The listing builds one solid part. Answer for the finished solid, in the listing's coordinates (mm). Give positions to 0.01 mm unless a question says otherwise; leave off trailing zeros. Loops run counter-clockwise (first coordinate to the right, second up) from the corner with the lowest first, then second, coordinate; pieces in that order, holes last.
Item 1: Section A-A, the plane z = 117.5 is taken. Give the vertices of the cut face in (x, y).
Item 2: Section B-B, the plane y = -10.5 is taken. Give the vertices of the cut face in (x, z).
Item 3: Consider line 1 along Z through (x, y) = (0, -4.75); line 2 along X through (y, z) = (3.5, 238). Determine where each line is inside the solid, lowest interval first.
Item 4: Each of these flat-tipped pins is pushed along its axis until it touches: pin 1 Ø2.5 at (x, y) = (0.5, -2) entering from -Z; pin 2 Ø5 at (x, y) = (10, -6) entering from -Z; pin 3 Ø1 at (x, y) = (1, -6) entering from +Z; pin 4 Ø3 at (x, z) = (0, 5) entering from +Y. Where does it stop, or does it pass through?
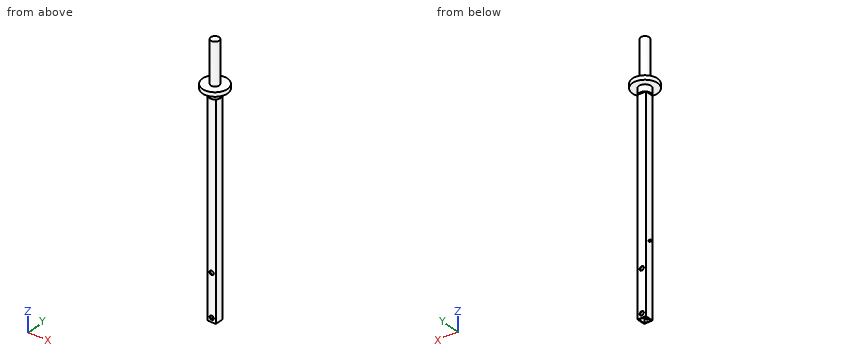
from build123d import *

# Parameters (mm, degrees)
SKETCH_W     = 10
SKETCH_H     = 10
SKETCH_W_2   = 8
SKETCH_H_2   = 8
PAD_DEPTH    = 250
SKETCH001_R  = 2.5
POCKET_DEPTH = 10.001
SKETCH002_R  = 1
PAD001_DEPTH = 2
SKETCH003_R  = 7.071068
PAD002_DEPTH = 8
SKETCH004_R  = 15
PAD003_DEPTH = 5
SKETCH005_R  = 5
PAD004_DEPTH = 50


with BuildPart() as part:
    # Sketch → Pad (new body)
    with BuildSketch(Plane.XY):
        Rectangle(SKETCH_W, SKETCH_H)
        Rectangle(SKETCH_W_2, SKETCH_H_2, mode=Mode.SUBTRACT)
    extrude(amount=PAD_DEPTH)

    # Sketch001 (on Face3 of Pad) → Pocket (cut, through all)
    with BuildSketch(Plane.XZ.offset(5)):
        with Locations((0, 5)):
            Circle(SKETCH001_R)
        with Locations((0, 55)):
            Circle(SKETCH001_R)
    extrude(amount=-POCKET_DEPTH, mode=Mode.SUBTRACT)

    # Sketch002 (on Face2 of Pocket) → Pad001 (join)
    with BuildSketch(Plane(origin=(-5, 0, 0), x_dir=(0, -1, 0), z_dir=(-1, 0, 0))):
        with Locations((0, 86)):
            Circle(SKETCH002_R)
    extrude(amount=PAD001_DEPTH)

    # Sketch003 (on Face4 of Pad001) → Pad002 (join)
    with BuildSketch(Plane.XY.offset(250)):
        Circle(SKETCH003_R)
    extrude(amount=PAD002_DEPTH)

    # Sketch004 (on Face6 of Pad002) → Pad003 (join)
    with BuildSketch(Plane.XY.offset(258)):
        Circle(SKETCH004_R)
    extrude(amount=PAD003_DEPTH)

    # Sketch005 (on Face3 of Pad003) → Pad004 (join)
    with BuildSketch(Plane.XY.offset(263)):
        Circle(SKETCH005_R)
    extrude(amount=PAD004_DEPTH)


solid = part.part
Worked answers:
1. outline: (-5, -5) - (5, -5) - (5, 5) - (-5, 5) - close; hole (-4, -4) - (4, -4) - (4, 4) - (-4, 4) - close
2. outline: (-10.71, 258) - (10.71, 258) - (10.71, 263) - (-10.71, 263) - close
3. line 1: z = 0 to 2.5, 7.5 to 52.5, 57.5 to 313
3. line 2: x = -5 to -4, 4 to 5
4. pin 1: stops at z = 250
4. pin 2: stops at z = 258
4. pin 3: stops at z = 263
4. pin 4: passes through
